Could you check a few things on this model? Use its own coordinates, in mm. A direction names the side the tool comes from. Give positions to 0.01 mm unless a question says otherwise; leave off trailing zeros. Loops run counter-clockwise (first coordinate to the right, second up) from the corner with the lowest first, then second, coordinate; pieces in that order, holes last. Notation, with made-up numbers: (43, -10.75) -> (73, -10.75) arc R27 cw to (73, 26.25) -> close; hole circle Ø2 at (-12, 11). An arc over 180 degrees is marked (long way). Write item = value, one per line. Start each with the question number.
1) I need wall thicknesses on probe 1 along Y at (x, z) = (-4.5, 70); probe 2 along Y at (x, z) = (-20, -7); probe 3 along X at (y, z) = (29, 10). Which ranges of each line are inside material? Lowest first, please. Write a range as from..to.
2) I want a section at D-D (z = 12). List the corners of the cut face in (x, y) for me, and give its area (3 significant figures).
3) I want a section at B-B (z = 0). List the corners of the cut face in (x, y) for me.
4) If we mould it in two halves opening along Z, with no side actions, what happens to faces 6 (the face through (0, 8, 79.75)), 7 (the face through (0, 15, 55)), 8 (the face through (-12.18, 36.05, 9.34))? For each: +Z half, -Z half, draft (parallel to the pull), parting line (faces both ways), or undercut.
5) I'm going to push flat-ended pins straight in: pin 1 Ø14 at (x, z) = (1.5, 51.5) entering from +Y; pin 2 Ø7.5 at (y, z) = (6, 60) entering from +X; pin 3 Ø10 at (x, y) = (-1, 22.5) entering from -Z. Where does each tip first touch, or does it pass through?
6) I want a section at A-A (x = 0). List the corners of the cut face in (y, z) for me, and give its area (3 significant figures).
7) On a 3-axis mill with a long thin cutter (end or side, diameter ignored), from which of +Z, -Z, +X, -X, +Y, -Y can I reach the whole of each face in a straight line? I mean faces 1 (the face through (6.4, 7, 55)), 2 (the face through (0, 43.3, 0)), 3 (the face through (0, 0, 1)), 4 (the face through (-7, 28.6, -14)), 5 (the face through (-6.4, 8, 55)). Say none if no direction works.
8) I want a section at C-C (y = 18). List the corners of the cut face in (x, z) for me.
Autodesk Inventor part; units mm, degrees
ref_plane "Work Plane1" through (0, 0, 30.75) normal (0, 0, 1) x (1, 0, 0)
ref_plane "YZ Plane" through (0, 0, 0) normal (1, 0, 0) x (0, 1, 0)
ref_plane "XZ Plane" through (0, 0, 0) normal (0, 1, 0) x (-1, 0, 0)
sketch "Sketch1" plane through (0, 0, 0) normal (0, 1, 0) x (-1, 0, 0)
  circle A0 centre (0, 0) radius 30.75
  dimension "d0" = 61.5
extrude "Extrusion1" add sketch "Sketch1" along normal blind 43.3
ref_plane "Work Plane1" through (0, 0, 30.75) normal (0, 0, 1) x (1, 0, 0)
sketch "Sketch2" plane through (0, 0, 30.75) normal (0, 0, 1) x (1, 0, 0)
  line L0 (30.75, 0) -> (-30.75, 0)
  line L1 (6.4, 15) -> (-6.4, 15)
  line L2 (-6.4, 15) -> (-6.4, 0)
  line L3 (-6.4, 0) -> (6.4, 0)
  line L4 (6.4, 0) -> (6.4, 15)
extrude "Extrusion2" add sketch "Sketch2" along normal blind 49
sketch "Sketch3" plane through (0, 0, 30.75) normal (0, 0, -1) x (-1, 0, 0)
  line L0 (6.4, 15) -> (6.4, 0)
  line L1 (-6.4, 0) -> (-6.4, 15)
  line L2 (6.4, 0) -> (-6.4, 0)
  line L3 (-6.4, 0) -> (-6.4, 15)
  line L4 (-6.4, 15) -> (6.4, 15)
  line L5 (6.4, 15) -> (6.4, 0)
  point P0 (0, 0)
extrude "Extrusion3" add sketch "Sketch3" along normal blind 5
sketch "Sketch4" plane through (0, 43.3, 0) normal (0, 1, 0) x (1, 0, 0)
  circle A0 centre (0, 0) radius 15.35
  circle A1 centre (0, 0) radius 30.75
  dimension "d10" = 30.7
extrude "Extrusion4" cut sketch "Sketch4" against normal blind 14.7
properties part number "Camara"
Answer list:
q1.probe_1 = 0..15
q1.probe_2 = 0..28.6
q1.probe_3 = -11.65..11.65
q2.outline = (-28.31, 0) -> (28.31, 0) -> (28.31, 28.6) -> (9.57, 28.6) -> (9.57, 43.3) -> (-9.57, 43.3) -> (-9.57, 28.6) -> (-28.31, 28.6) -> close
q2.area = 1,900 mm^2
q3.outline = (-30.75, 0) -> (30.75, 0) -> (30.75, 28.6) -> (15.35, 28.6) -> (15.35, 43.3) -> (-15.35, 43.3) -> (-15.35, 28.6) -> (-30.75, 28.6) -> close
q4.face_6 = +Z half
q4.face_7 = draft
q4.face_8 = parting line
q5.pin_1 = 15
q5.pin_2 = 6.4
q5.pin_3 = -30.75
q6.outline = (0, -30.75) -> (28.6, -30.75) -> (28.6, -15.35) -> (43.3, -15.35) -> (43.3, 15.35) -> (28.6, 15.35) -> (28.6, 30.75) -> (15, 30.75) -> (15, 79.75) -> (0, 79.75) -> close
q6.area = 2,950 mm^2
q7.face_1 = +Z, +X, +Y, -Y
q7.face_2 = +Z, -Z, +X, -X, +Y
q7.face_3 = +Z, -Z, +X, -X, -Y
q7.face_4 = +Y
q7.face_5 = +Z, -X, +Y, -Y
q8.outline = circle Ø61.5 at (0, 0)
